Autodesk Inventor part; units mm, degrees
ref_plane "YZ Plane" through (0, 0, 0) normal (1, 0, 0) x (0, 1, 0)
ref_plane "XZ Plane" through (0, 0, 0) normal (0, 1, 0) x (-1, 0, 0)
ref_plane "XY Plane" through (0, 0, 0) normal (0, 0, 1) x (1, 0, 0)
sketch "Sketch1" plane through (0, 0, 0) normal (0, 1, 0) x (-1, 0, 0)
  circle A0 centre (0, 0) radius 2.63
  line L0 (0, 0) -> (0, -2.63) construction
  line L1 (0, 0) -> (2.63, 0) construction
  circle A1 centre (20, 0) radius 2.63
  circle A2 centre (0, -10) radius 1.35
  circle A3 centre (-9.525, -10) radius 1.35
  circle A4 centre (20, 0) radius 5.805 construction
  circle A5 centre (0, 0) radius 5.805 construction
  circle A6 centre (0, -10) radius 4.525 construction
  circle A7 centre (-9.525, -10) radius 4.525 construction
  line L2 (-4.5564, 3.5969) -> (-13.0767, -7.1962)
  line L3 (22.2946, -5.3322) -> (1.7886, -14.1565)
  line L4 (20, 5.805) -> (0, 5.805)
  line L5 (0, -14.525) -> (-9.525, -14.525)
  arc A8 (22.2946, -5.3322) -> (20, 5.805) centre (20, 0) ccw
  arc A9 (0, 5.805) -> (-4.5564, 3.5969) centre (0, 0) ccw
  arc A10 (0, -14.525) -> (1.7886, -14.1565) centre (0, -10) ccw
  arc A11 (-13.0767, -7.1962) -> (-9.525, -14.525) centre (-9.525, -10) ccw
  point P0 (-13.5097, -12.8558)
  dimension "d0" = 5.26
  dimension "d1" = 20
  dimension "d2" = 2.7
  dimension "d3" = 10
  dimension "d4" = 9.525
  dimension "d5" = 3.175
  dimension "d6" = 3.175
extrude "Extrusion1" add sketch "Sketch1" along normal blind 4
sketch "Sketch2" plane through (0, 0, 0) normal (0, -1, 0) x (1, 0, 0)
  line L0 (-20, 5.805) -> (0, 5.805)
  arc A0 (-20, 5.805) -> (-22.2946, -5.3322) centre (-20, 0) ccw
  line L1 (-1.7886, -14.1565) -> (-22.2946, -5.3322)
  arc A1 (-1.7886, -14.1565) -> (0, -14.525) centre (0, -10) ccw
  line L2 (9.525, -14.525) -> (0, -14.525)
  arc A2 (9.525, -14.525) -> (13.0767, -7.1962) centre (9.525, -10) ccw
  line L3 (4.5564, 3.5969) -> (13.0767, -7.1962)
  arc A3 (4.5564, 3.5969) -> (0, 5.805) centre (0, 0) ccw
  circle A4 centre (-20, 0) radius 2.63
  circle A5 centre (9.525, -10) radius 1.35
  circle A6 centre (0, -10) radius 1.35
  circle A7 centre (0, 0) radius 2.63
  circle A8 centre (9.525, -10) radius 2
  circle A9 centre (0, -10) radius 2
  dimension "d9" = 4
extrude "Extrusion2" cut sketch "Sketch2" against normal blind 2.5 contours A8 | A9
chamfer "Chamfer1" distance 0.7937 angle 45 8 edges at (-10, 4, 5.805) (2.5316, 4, 5.2239) (8.8165, 4, -1.7997) (13.597, 4, -11.9734) (4.7625, 4, -14.525) (-0.9131, 4, -14.4319) (-12.0416, 4, -9.7444) (-25.6856, 4, 1.1714)
properties part number "CNC-010-XAxisLimitSwitchMount" material "ABS Plastic"
Could you check a few things on this model? Use its own coordinates, in mm. A direction names the side the tool comes from. Round coordinates to 2 decimals unless told otherwise and drop trailing zeros. Loops run counter-clockwise (first coordinate to the right, second up) from the corner with the lowest first, then second, coordinate; pieces in that order, holes last. Notation, with made-up numbers: (-22, 41.5) - (3, 41.5) arc R7 ccw to (3, 45.5) - close; hole circle Ø5 at (42, -15). An arc over 180 degrees is marked (long way). Answer in a Markdown table with one row per item. Add a question column.
(1) I'm going to push flat-ended pins straight in: pin 1 (4 mm diameter, centred on x = 0, z = 0, fed in from +Y); pin 2 (3 mm diameter, centred on x = 0, z = -10, fed in from -Y); pin 3 (2 mm diameter, centred on y = 1.5, z = -6.5, fed in from -X). Where does each tip first touch, or does it pass through?
(2) If we section it at C-C (x = -17): Please give me the cut outline in (y, z) (3 decimals).
(3) For faces 1 (the face through (-0.93, 1.58, -14.43)), 2 (the face through (9.265, 1.232, -8.017)), which set-ups out of +Z, -Z, +X, -X, +Y, -Y let a thin tool reach every point of the face, with its end or its side?
(4) If we mould it in two halves opening along Z, with no side actions, what happens to faces 3 (the face through (-12.19, 1.58, -9.68)), 4 (the face through (8, 2.5, -10)), 5 (the face through (-25.662, 1.581, 1.28))? For each: pulls with the +Z half, pulls with the -Z half, needs draft (parallel to the pull), parting line crosses it, or undercut.
(5) I need wall thicknesses on line 1 along Z through (x, y) = (0, 1.8) (3 decimals); line 2 along Z through (x, y) = (9, 1.2) (3 decimals); line 3 along X through (y, z) = (1.7, 0.75). Which ranges of each line are inside material? Lowest first, please.
(6) If we section it at A-A (y = 0.4): State how many separate pieces and enclosed holes the cut face has, plus the area to 3 significant figures.
Model answer:
| question | item | result |
|---|---|---|
| 1 | pin 1 | passes through |
| 1 | pin 2 | stops at y = 2.5 |
| 1 | pin 3 | stops at x = -21.9 |
| 2 | outline | (0, -7.611) - (3.206, -7.611) - (4, -6.747) - (4, 5.011) - (3.206, 5.805) - (0, 5.805) - close |
| 3 | face 1 | -Z, -X, +Y, -Y |
| 3 | face 2 | -Y |
| 4 | face 3 | pulls with the -Z half |
| 4 | face 4 | undercut |
| 4 | face 5 | parting line crosses it |
| 5 | line 1 | z = -14.525 to -12, -8 to -2.63, 2.63 to 5.805 |
| 5 | line 2 | z = -14.525 to -11.93, -8.07 to -2.032 |
| 5 | line 3 | x = -25.76 to -22.52, -17.48 to -2.52, 2.52 to 6.8 |
| 6 | separate pieces | 1 |
| 6 | enclosed holes | 4 |
| 6 | area | 513 mm² |
